CAD build for the part. Positions are in the model's coordinates, mm. A direction names the side the tool comes from. Round coordinates to 2 decimals unless told otherwise and drop trailing zeros. Loops run counter-clockwise (first coordinate to the right, second up) from the corner with the lowest first, then second, coordinate; pieces in that order, holes last. Notation, with made-up numbers: M 60,-16 L 86,-16 A32 cw 86,11 Z; hole C 67.25,-12 d9. An arc over 180 degrees is marked long. Use a Markdown table: item, result. Add a question column.
(1) Wall check: L1, parallel to Y at x = 0.3, z = -1.5; L2, parallel to X at y = 1.5, z = -0.25; L3, parallel to Z at x = 0.25, y = 0.35. Give the ranges that are in metal, low to high.
(2) Band-saw the part on A-A, the plane y = 0.5. Write the cut outline in (x, z), and give its area (3 significant figures).
(3) Band-saw the part on C-C, the plane x = 3.6. Write the cut outline in (y, z).
(4) Band-saw the part on B-B, the plane z = 2. Write the cut outline in (x, y).
(5) Which spindle directions (+Z, -Z, +X, -X, +Y, -Y) get a long thin tool onto all of the face, cutting with end or side? Do faces 1 (the face through (0.3, 0, 3.7)), 2 (the face through (1.932, -0.189, 3.188)). Say none if no direction does.
(6) Band-saw the part on D-D, the plane z = -0.25. Write the cut outline in (x, y).
(7) Flat gauge pins, fed straight in: P1, Ø1, axis at x = 2, z = -1, coming from the -Y side; P2, Ø1.5, axis at x = 2.5, y = -1.5, coming from the +Z side; P3, Ø0.8, axis at x = 3.5, z = 2, coming from the -Y side. Where does each tip first touch, or does it go through?
from build123d import *

# Parameters (mm, degrees)
F0_W     = 3.9
F0_H     = 3.5
F1_DEPTH = 0.7
F2_R     = 1.45
F3_DEPTH = 3.2
F5_DEPTH = 1
F6_SIZE  = 0.3
F8_DEPTH = 0.7


with BuildPart() as f1:
    # F0 (on Right) → F1 (new body)
    with BuildSketch(Plane.YZ):
        Rectangle(F0_W, F0_H)
        with BuildLine():
            Line((-1.95, 1.75), (1.95, 1.75))
            ThreePointArc((1.95, 1.75), (0, 3.7), (-1.95, 1.75))
        make_face()
        with BuildLine():
            ThreePointArc((-1.95, -1.75), (0, -3.7), (1.95, -1.75))
            Line((1.95, -1.75), (-1.95, -1.75))
        make_face()
    extrude(amount=F1_DEPTH)

    # F2 (on Right) → F3 (join)
    with BuildSketch(Plane.YZ):
        with Locations((0, 1.75)):
            Circle(F2_R)
    extrude(amount=F3_DEPTH)

    # F4 (on face) → F5 (join)
    with BuildSketch(Plane.YZ.offset(3.2)):
        Polygon((1.05, 1.143782), (1.05, 2.356218), (0, 2.962436), (-1.05, 2.356218), (-1.05, 1.143782), (0, 0.537564), align=None)
    extrude(amount=F5_DEPTH)

    # F6
    f6_edges = [f1.edges().sort_by_distance(p)[0] for p in [
        (4.2, -0.525, 2.659327),
        (4.2, 0.525, 2.659327),
        (4.2, 1.05, 1.75),
        (4.2, 0.525, 0.840673),
        (4.2, -0.525, 0.840673),
        (4.2, -1.05, 1.75),
    ]]
    chamfer(f6_edges, length=F6_SIZE)

    # F7 (on face) → F8 (cut, through all)
    with BuildSketch(Plane(origin=(0, 0, 0), x_dir=(0, -1, 0), z_dir=(-1, 0, 0))):
        Polygon((1.1, -2.385085), (1.1, -1.114915), (0, -0.479829), (-1.1, -1.114915), (-1.1, -2.385085), (0, -3.020171), align=None)
    extrude(amount=-F8_DEPTH, mode=Mode.SUBTRACT)


solid = f1.part
Return value:
| question | item | result |
|---|---|---|
| 1 | L1 | -1.95 to -1.1, 1.1 to 1.95 |
| 1 | L2 | 0 to 0.7 |
| 1 | L3 | -3.67 to -2.82, -0.68 to 3.67 |
| 2 | outline | M 0,-3.63 L 0.7,-3.63 L 0.7,-2.73 L 0,-2.73 Z; M 0,-0.77 L 0.7,-0.77 L 0.7,0.39 L 3.2,0.39 L 3.2,0.83 L 3.9,0.83 L 4.2,1.17 L 4.2,2.33 L 3.9,2.67 L 3.2,2.67 L 3.2,3.11 L 0.7,3.11 L 0.7,3.63 L 0,3.63 Z |
| 2 | area | 12.3 mm^2 |
| 3 | outline | M -1.05,1.14 L 0,0.54 L 1.05,1.14 L 1.05,2.36 L 0,2.96 L -1.05,2.36 Z |
| 4 | outline | M 0,-1.93 L 0.7,-1.93 L 0.7,-1.43 L 3.2,-1.43 L 3.2,-1.05 L 3.9,-1.05 L 4.2,-0.75 L 4.2,0.75 L 3.9,1.05 L 3.2,1.05 L 3.2,1.43 L 0.7,1.43 L 0.7,1.93 L 0,1.93 Z |
| 5 | face 1 | +Z, +X, -X |
| 5 | face 2 | +X |
| 6 | outline | M 0,-1.95 L 0.7,-1.95 L 0.7,1.95 L 0,1.95 Z |
| 7 | P1 | through |
| 7 | P2 | z = 2.99 |
| 7 | P3 | y = -1.45 |
